from build123d import *

# Parameters (mm, degrees)
F0_R     = 50.8
F0_W     = 19.494822
F0_H     = 11.168908
F0_R_2   = 12.7
F0_W_2   = 17.667183
F0_H_2   = 11.16891
F1_DEPTH = 6.35


with BuildPart() as f1:
    # F0 (on Top) → F1 (new body, symmetric)
    with BuildSketch(Plane.XY):
        Circle(F0_R)
        with Locations((-2.842995, -34.623617)):
            Rectangle(F0_W, F0_H, mode=Mode.SUBTRACT)
        Circle(F0_R_2, mode=Mode.SUBTRACT)
        with Locations((17.362575, 25.48542)):
            Rectangle(F0_W_2, F0_H_2, mode=Mode.SUBTRACT)
    extrude(amount=F1_DEPTH, both=True)


solid = f1.part
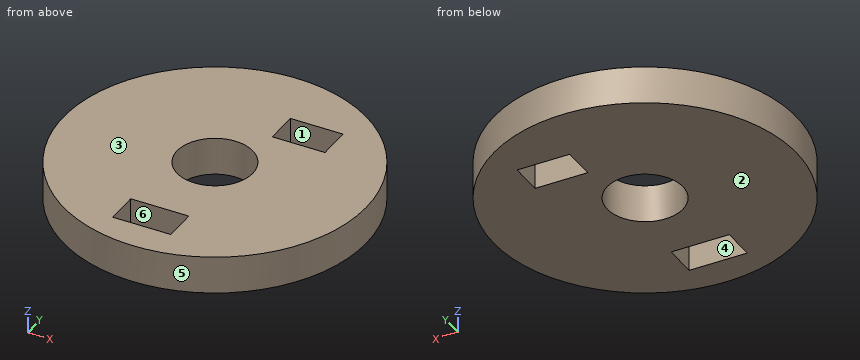
Check sheet for the modelled part. Datum: model origin and axes. Units: mm. Face numbers are marked on the shaded views. A direction names the side the tool comes from. Round coordinates to 2 decimals unless told otherwise and drop trailing zeros. Write each loop counter-clockwise with the first axis right and the second up, starting at its lowest first coordinate (ties: lowest second). Pieces come first, ordered by that corner, then holes. Notation, with made-up numbers: (21, 27) - (64, 27) arc R29 ccw to (64, 66) - close; hole circle Ø5 at (-21, -11.75). An arc over 180 degrees is marked (long way). Return JSON: item names as keys, results as strings.
Q1. Access from +Z, -Z, +X, -X, +Y, -Y to the whole of each face (thin tool, end or side, straight path). Record for the marked faces 1 and 2.
Returned:
{"face 1": "+Z, -Z", "face 2": "-Z, +X, -X, +Y, -Y"}
Q2. Cross-section at B-B (x = 0). Record the boundary of the cut face in (y, z).
Returned:
{"outline": "(-50.8, -6.35) - (-40.21, -6.35) - (-40.21, 6.35) - (-50.8, 6.35) - close; (-29.04, -6.35) - (-12.7, -6.35) - (-12.7, 6.35) - (-29.04, 6.35) - close; (12.7, -6.35) - (50.8, -6.35) - (50.8, 6.35) - (12.7, 6.35) - close"}
Q3. Scan lines: L1, parallel to Y at x = 0, z = -1; L2, parallel to Y at x = 9.5, z = 2; L3, parallel to X at y = 5, z = -3.75. Record each from-to range of solid material in increasing order. Write a range as from..to.
Returned:
{"L1": "y = -50.8..-40.21, -29.04..-12.7, 12.7..50.8", "L2": "y = -49.9..-8.43, 8.43..19.9, 31.07..49.9", "L3": "x = -50.55..-11.67, 11.67..50.55"}
Q4. Cross-section at A-A (y = 0). Record the boundary of the cut face in (x, z).
Returned:
{"outline": "(-50.8, -6.35) - (-12.7, -6.35) - (-12.7, 6.35) - (-50.8, 6.35) - close; (12.7, -6.35) - (50.8, -6.35) - (50.8, 6.35) - (12.7, 6.35) - close"}
Q5. Cross-section at C-C (z = 0). Record the boundary of the cut face in (x, y).
Returned:
{"outline": "circle Ø101.6 at (0, 0); hole circle Ø25.4 at (0, 0); hole (-12.59, -40.21) - (6.9, -40.21) - (6.9, -29.04) - (-12.59, -29.04) - close; hole (8.53, 19.9) - (26.2, 19.9) - (26.2, 31.07) - (8.53, 31.07) - close"}
Q6. Draft check along Y on the marked faces 3, 4, 5 and 6. Enter one of: released by +Y, released by -Y, zero draft, split by the parting line, or undercut.
Returned:
{"face 3": "zero draft", "face 4": "undercut", "face 5": "split by the parting line", "face 6": "undercut"}
Q7. Depth check by flat-ended pin: P1, Ø2, axis at x = 24, z = 3.5, coming from the +Y side; P2, Ø2, axis at x = 31.5, z = 4, coming from the +Y side (3 decimals); P3, Ø1, axis at x = -29.5, z = -1.5, coming from the +Y side. Enter the tip coordinate at first touch or a pass-through.
Returned:
{"P1": "stops at y = 45.3", "P2": "stops at y = 40.625", "P3": "stops at y = 41.71"}
Q8. Cross-section at D-D (x = 20.5). Record the boundary of the cut face in (y, z).
Returned:
{"outline": "(-46.48, -6.35) - (19.9, -6.35) - (19.9, 6.35) - (-46.48, 6.35) - close; (31.07, -6.35) - (46.48, -6.35) - (46.48, 6.35) - (31.07, 6.35) - close"}
